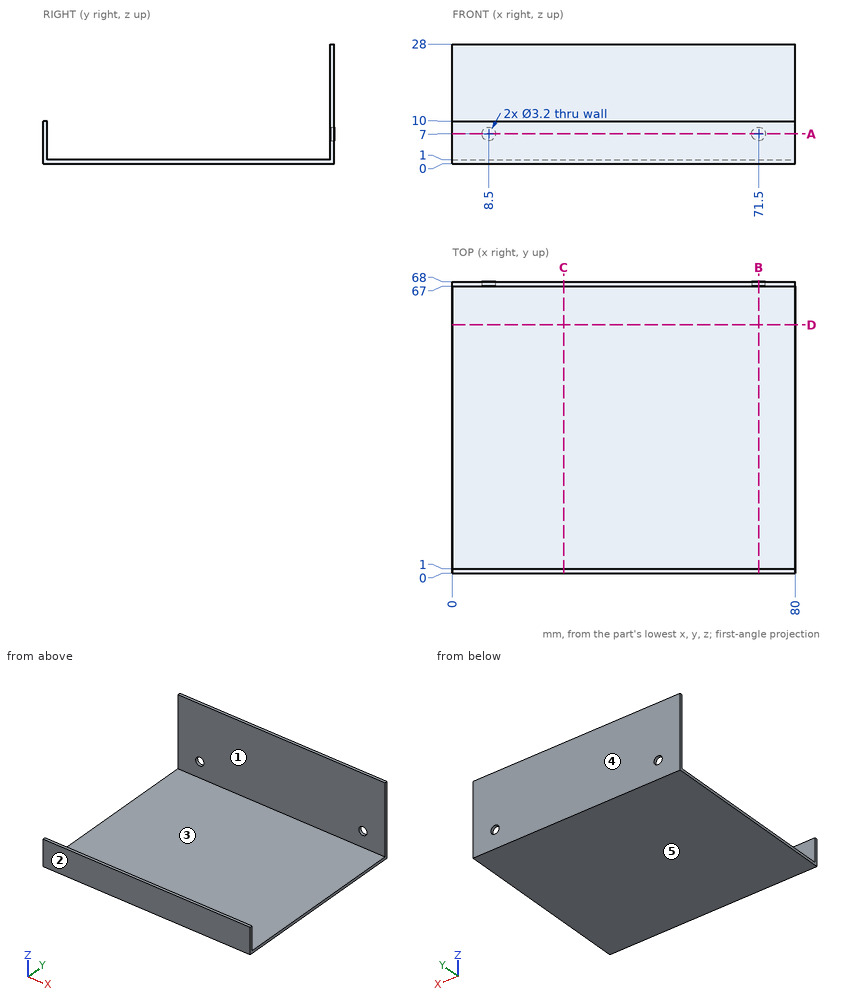
Part print with two shaded views. Sizes in mm from the minimum x, y, z corner. A direction names the side the tool comes from. Round coordinates to 2 decimals unless told otherwise and drop trailing zeros. Order: outer loops, then holes, each group sorted by start corner. A loop starts at its lowest first (then second) coordinate and runs counter-clockwise, first axis right, second up. Notation, with made-up numbers: (-8, -35) - (47, -35) arc R31 cw to (47, 1) - close; hole circle Ø6 at (58, 17). An arc over 180 degrees is marked (long way). Answer in a Markdown table with one row per item. Add a question column.
(1) Band-saw the part on A-A on z = 7. List the corners of the cut face in (x, y).
(2) Band-saw the part on C-C on x = 26. List the corners of the cut face in (y, z).
(3) Probe L1, parallel to Z at x = 71.5, y = 67.6; L2, parallel to Y at x = 47, z = 6.25; L3, parallel to Y at x = 8, z = 23.75. List the from-to ranges inside material, lowest first. Write a range as [from, to].
(4) Mould opens along Y. For the marked faces 3, 4 and 5 say: +Y half, -Y half, draft (parallel to the pull), parting line (faces both ways), or undercut.
(5) Band-saw the part on D-D on y = 58. List the corners of the cut face in (x, z), and give its area (3 significant figures).
(6) Drop flat-ended pins along their axis: pin 1 Ø12 at (x, y) = (27.5, 9) entering from +Z; pin 2 Ø1.9 at (x, z) = (71.5, 7) entering from +Y; pin 3 Ø1.1 at (x, y) = (35.5, 0.5) entering from +Z; pin 4 Ø3.5 at (x, z) = (8.5, 7) entering from -Y. Give the stop position or say it passes through.
(7) 3-axis set-ups, long thin cutter, end or side, ignore diameter. For the marked faces 1 and 2: which of +Z, -Z, +X, -X, +Y, -Y reach the whole face in a straight line?
(8) Band-saw the part on B-B on x = 71.5. List the corners of the cut face in (y, z).
Data:
| question | item | result |
|---|---|---|
| 1 | outline | (0, 0) - (80, 0) - (80, 1) - (0, 1) - close; (0, 67) - (6.9, 67) - (6.9, 68) - (0, 68) - close; (10.1, 67) - (69.9, 67) - (69.9, 68) - (10.1, 68) - close; (73.1, 67) - (80, 67) - (80, 68) - (73.1, 68) - close |
| 2 | outline | (0, 0) - (68, 0) - (68, 28) - (67, 28) - (67, 1) - (1, 1) - (1, 10) - (0, 10) - close |
| 3 | L1 | z = [0, 5.4], [8.6, 28] |
| 3 | L2 | y = [0, 1], [67, 68] |
| 3 | L3 | y = [67, 68] |
| 4 | face 3 | undercut |
| 4 | face 4 | +Y half |
| 4 | face 5 | draft |
| 5 | outline | (0, 0) - (80, 0) - (80, 1) - (0, 1) - close |
| 5 | area | 80.0 mm^2 |
| 6 | pin 1 | stops at z = 1 |
| 6 | pin 2 | stops at y = 1 |
| 6 | pin 3 | stops at z = 10 |
| 6 | pin 4 | stops at y = 0 |
| 7 | face 1 | +Z, +X, -X |
| 7 | face 2 | +Z, -Z, +X, -X, -Y |
| 8 | outline | (0, 0) - (68, 0) - (68, 5.4) - (67, 5.4) - (67, 1) - (1, 1) - (1, 10) - (0, 10) - close; (67, 8.6) - (68, 8.6) - (68, 28) - (67, 28) - close |
